Geometry check sheet. Reference: the model listing, model coordinates, mm. A direction names the side the tool comes from. Round coordinates to 2 decimals unless told otherwise and drop trailing zeros. Order: outer loops, then holes, each group sorted by start corner. A loop starts at its lowest first (then second) coordinate and runs counter-clockwise, first axis right, second up.
(1) Cross-section at A-A on z = 0. Enter the section's corners in (x, y).
(2) Set-up check for faces 1 (the face through (0, 0, 0)), 2 (the face through (70, 7, 0)): record each of +Z, -Z, +X, -X, +Y, -Y from which the full face is reachable in a straight line by a thin tool's end or side.
(3) Draft check along X on faces 3 (the face through (98.61, -9.76, 2.17)), 4 (the face through (200, 0, 0)), 5 (the face through (130, 7, 0)). Enter one of: pulls with the +X half, pulls with the -X half, needs draft (parallel to the pull), parting line crosses it, or undercut.
(4) Cross-section at B-B on x = 28. Enter the section's corners in (y, z).
(5) Gauge pin test, flat ends, axial feed: P1, Ø3, axis at x = 129, y = 9, coming from the +Z side; P2, Ø2, axis at x = 72.5, y = 8, coming from the +Z side; P3, Ø2, axis at x = 23, z = 3, coming from the +Y side. Record the tip position at first contact, or that the pin passes through.
(6) Thickness scan on L1, parallel to Y at x = 150, z = 0.25; L2, parallel to Z at x = 42.5, y = -3; L3, parallel to X at y = -4.75, z = 8.25. Record the ranges inside material, lowest first.
from build123d import *

# Parameters (mm, degrees)
SKETCH_1_R          = 10
EXTRUDE_1_DEPTH     = 100
CUT_EXTRUDE_1_DEPTH = 3
CHAMFER_1_SIZE      = 0.5
SKETCH_3_R          = 10
EXTRUDE_2_DEPTH     = 100
CUT_EXTRUDE_2_DEPTH = 3
CHAMFER_2_SIZE      = 0.5


with BuildPart() as part:
    # 草图1 → 凸台-拉伸1 (new body)
    with BuildSketch(Plane(origin=(0, 0, 0), x_dir=(0, 0, -1), z_dir=(1, 0, 0))):
        Circle(SKETCH_1_R)
    extrude(amount=EXTRUDE_1_DEPTH)

    # 草图2 → 切除-拉伸1 (cut)
    with BuildSketch(Plane(origin=(0, 10, 0), x_dir=(1, 0, 0), z_dir=(0, 1, 0))):
        with BuildLine():
            Line((63, 3), (77, 3))
            ThreePointArc((77, 3), (80, 0), (77, -3))
            Line((77, -3), (63, -3))
            ThreePointArc((63, -3), (60, 0), (63, 3))
        make_face()
    extrude(amount=-CUT_EXTRUDE_1_DEPTH, mode=Mode.SUBTRACT)

    # 倒角1
    chamfer_1_edges = [part.edges().sort_by_distance(p)[0] for p in [
        (0, 0, 10),
    ]]
    chamfer(chamfer_1_edges, length=CHAMFER_1_SIZE)

    # 草图3 → 凸台-拉伸2 (add)
    with BuildSketch(Plane(origin=(100, 0, 0), x_dir=(0, 0, -1), z_dir=(1, 0, 0))):
        Circle(SKETCH_3_R)
    extrude(amount=EXTRUDE_2_DEPTH)

    # 草图4 → 切除-拉伸2 (cut)
    with BuildSketch(Plane(origin=(0, 10, 0), x_dir=(1, 0, 0), z_dir=(0, 1, 0))):
        with BuildLine():
            Line((123, 3), (137, 3))
            ThreePointArc((137, 3), (140, 0), (137, -3))
            Line((137, -3), (123, -3))
            ThreePointArc((123, -3), (120, 0), (123, 3))
        make_face()
    extrude(amount=-CUT_EXTRUDE_2_DEPTH, mode=Mode.SUBTRACT)

    # 倒角2
    chamfer_2_edges = [part.edges().sort_by_distance(p)[0] for p in [
        (200, 0, 10),
    ]]
    chamfer(chamfer_2_edges, length=CHAMFER_2_SIZE)


solid = part.part
Found:
1. outline: (0, -9.5) - (0.5, -10) - (199.5, -10) - (200, -9.5) - (200, 9.5) - (199.5, 10) - (140, 10) - (140, 7) - (120, 7) - (120, 10) - (80, 10) - (80, 7) - (60, 7) - (60, 10) - (0.5, 10) - (0, 9.5) - close
2. face 1: +Z, -Z, -X, +Y, -Y
2. face 2: +Y
3. face 3: needs draft
3. face 4: pulls with the +X half
3. face 5: undercut
4. outline: circle Ø20 at (0, 0)
5. P1: stops at z = 6.61
5. P2: stops at z = 7.14
5. P3: stops at y = 9.8
6. L1: y = -10 to 10
6. L2: z = -9.54 to 9.54
6. L3: x = 0.02 to 199.98
